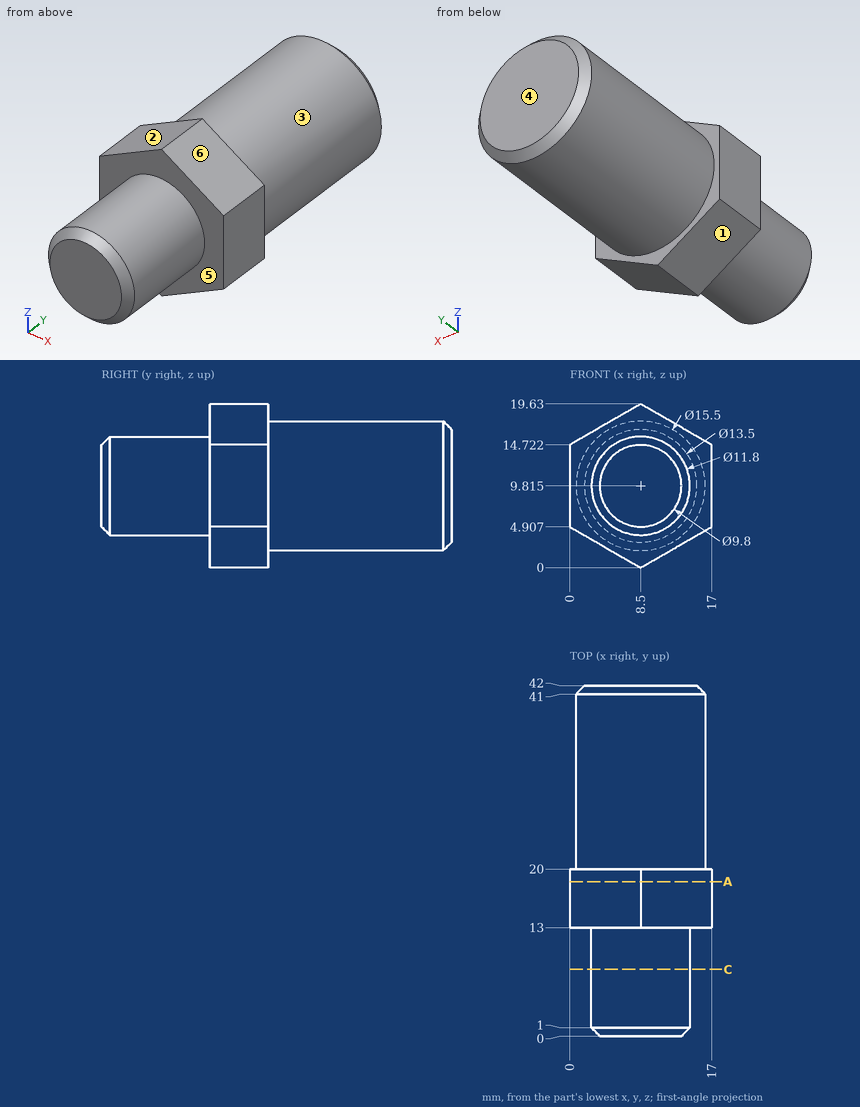
Part print with two shaded views. Sizes in mm from the minimum x, y, z corner. A direction names the side the tool comes from. Coordinates: 2 decimals unless noted, no trailing zeros. Write each loop counter-clockwise with the first axis right and the second up, starting at its lowest first coordinate (ties: lowest second). Pieces come first, ordered by that corner, then holes. Notation, with made-up numbers: (-24.75, -18) - (13.25, -18) arc R23 ccw to (13.25, 6) - close; hole circle Ø10 at (39, -20.75). An arc over 180 degrees is marked (long way). One line per item, written item: value. Start each with the question number.
1. Probe line 1 (Y direction, x = 2, z = 8.75); line 2 (Y direction, x = 15.25, z = 4.5); line 3 (X direction, y = 40, z = 7.75). List the from-to ranges inside material, lowest first. Write a range as from..to.
2. Flat gauge pins, fed straight in: pin 1 (2 mm diameter, centred on y = 11.5, z = 11.5, fed in from +X); pin 2 (3 mm diameter, centred on x = 6, y = 15.5, fed in from +Z); pin 3 (3 mm diameter, centred on y = 7, z = 3.5, fed in from +X). Where does each tip first touch, or does it go through?
3. Slice it at C-C (y = 8). Write the cut outline in (x, z) (1 decimal).
4. Tool access for the marked faces 5 and 6: list every direction of +Z, -Z, +X, -X, +Y, -Y with a clear straight run to the whole face (end or side of a thin tool).
5. Mould opens along Z. For the marked faces 1, 2, 3 and 4 say: released by +Z, released by -Z, zero draft, split by the parting line, or undercut.
6. Slice it at A-A (y = 18.5). Write the cut outline in (x, z), plus the area to 3 significant figures.
Answers below:
1. line 1: y = 13..42
1. line 2: y = 13..20
1. line 3: x = 1.03..15.97
2. pin 1: stops at x = 14.36
2. pin 2: stops at z = 19.05
2. pin 3: stops at x = 11.91
3. outline: circle Ø11.8 at (8.5, 9.8)
4. face 5: -Y
4. face 6: +Z, +X, +Y, -Y
5. face 1: released by -Z
5. face 2: released by +Z
5. face 3: split by the parting line
5. face 4: zero draft
6. outline: (0, 4.91) - (8.5, 0) - (17, 4.91) - (17, 14.72) - (8.5, 19.63) - (0, 14.72) - close
6. area: 250 mm^2
